```python
from build123d import *

# Parameters (mm, degrees)
F1_DEPTH = 10


with BuildPart() as f1:
    # F0 (on Front) → F1 (new body)
    with BuildSketch(Plane.XZ):
        with BuildLine():
            Line((0, 187.580806), (-550, 187.580806))
            ThreePointArc((-550, 187.580806), (-550.791112, 187.452333), (-551.500916, 187.080119))
            Line((-551.500916, 187.080119), (-582.495395, -144.660237))
            ThreePointArc((-582.495395, -144.660237), (-581.860029, -146.593552), (-580, -147.419194))
            Line((-580, -147.419194), (-6.159987, -147.419194))
            Line((-6.159987, -147.419194), (6.159987, -147.419194))
            Line((6.159987, -147.419194), (580, -147.419194))
            ThreePointArc((580, -147.419194), (581.860029, -146.593552), (582.495395, -144.660237))
            Line((582.495395, -144.660237), (551.500916, 187.080119))
            ThreePointArc((551.500916, 187.080119), (550.791112, 187.452333), (550, 187.580806))
            Line((550, 187.580806), (0, 187.580806))
        make_face()
        with BuildLine():
            ThreePointArc((-549.85201, 184.760109), (-549.012853, 185.366442), (-548, 185.580806))
            Line((-548, 185.580806), (0, 185.580806))
            Line((0, 185.580806), (548, 185.580806))
            ThreePointArc((548, 185.580806), (549.012853, 185.366442), (549.85201, 184.760109))
            Line((549.85201, 184.760109), (580.495395, -142.767521))
            ThreePointArc((580.495395, -142.767521), (579.820602, -144.632497), (578, -145.419194))
            Line((578, -145.419194), (0, -145.419194))
            Line((0, -145.419194), (-578, -145.419194))
            ThreePointArc((-578, -145.419194), (-579.820602, -144.632497), (-580.495395, -142.767521))
            Line((-580.495395, -142.767521), (-549.85201, 184.760109))
        make_face(mode=Mode.SUBTRACT)
    extrude(amount=F1_DEPTH)


solid = f1.part
```
Input: part model. Units: mm. Frame: model coordinates. Coordinates: 2 decimals unless noted, no trailing zeros. Write each loop counter-clockwise with the first axis right and the second up, starting at its lowest first coordinate (ties: lowest second). Pieces come first, ordered by that corner, then holes.
1) Section B-B on z = -26. Output: boundary loops of the cut face in (x, y), and give its area (3 significant figures).
2) Pin query (flat end, axial travel): pin 1 Ø1 at (y, z) = (-2.5, 23.5) entering from -X; pin 2 Ø5 at (y, z) = (-7.5, 66.5) entering from +X; pin 3 Ø1 at (y, z) = (-8.5, 84.5) entering from -X. Return the tip coordinate at first contact, or that it passes through.
3) Section A-A on x = 238. Output: boundary loops of the cut face in (y, z), and give its area (3 significant figures).
4) Mould query, pull axis X, two halves, no side actions, for faces 1 (the flat face through (-566.78, -4.93, 23.53)), 2 (the flat face through (567.215, -4.93, 18.888)), 3 (the flat face through (-565.39, -4.93, 18.7)). Classes: pulls with the +X half, pulls with the -X half, needs draft (parallel to the pull), parting line crosses it, or undercut.
5) Material intervals for line 1 along Z through (x, y) = (535, -5); line 2 along X through (y, z) = (-1.25, -133.5); line 3 along X through (y, z) = (-3.25, -16.5), sorted ascending.
6) Section C-C on y = -4.5. Output: boundary loops of the cut face in (x, z).
Check result:
1. outline: (-571.41, -10) - (-569.57, -10) - (-569.57, 0) - (-571.41, 0) - close; (569.57, -10) - (571.41, -10) - (571.41, 0) - (569.57, 0) - close
1. area: 36.8 mm2
2. pin 1: stops at x = -566.83
2. pin 2: stops at x = 563
2. pin 3: stops at x = -561.13
3. outline: (-10, -147.42) - (0, -147.42) - (0, -145.42) - (-10, -145.42) - close; (-10, 185.58) - (0, 185.58) - (0, 187.58) - (-10, 187.58) - close
3. area: 40.0 mm2
4. face 1: pulls with the -X half
4. face 2: pulls with the +X half
4. face 3: undercut
5. line 1: z = -147.42 to -145.42, 185.58 to 187.58
5. line 2: x = -581.45 to -579.63, 579.63 to 581.45
5. line 3: x = -570.52 to -568.68, 568.68 to 570.52
6. outline: (-582.5, -144.66) arc R2.51 ccw to (-580, -147.42) - (580, -147.42) arc R2.51 ccw to (582.5, -144.66) - (551.5, 187.08) arc R2.5 ccw to (550, 187.58) - (-550, 187.58) arc R2.5 ccw to (-551.5, 187.08) - close; hole (-580.5, -142.77) arc R2.5 ccw to (-578, -145.42) - (578, -145.42) arc R2.5 ccw to (580.5, -142.77) - (549.85, 184.76) arc R2.5 ccw to (548, 185.58) - (-548, 185.58) arc R2.5 ccw to (-549.85, 184.76) - close
